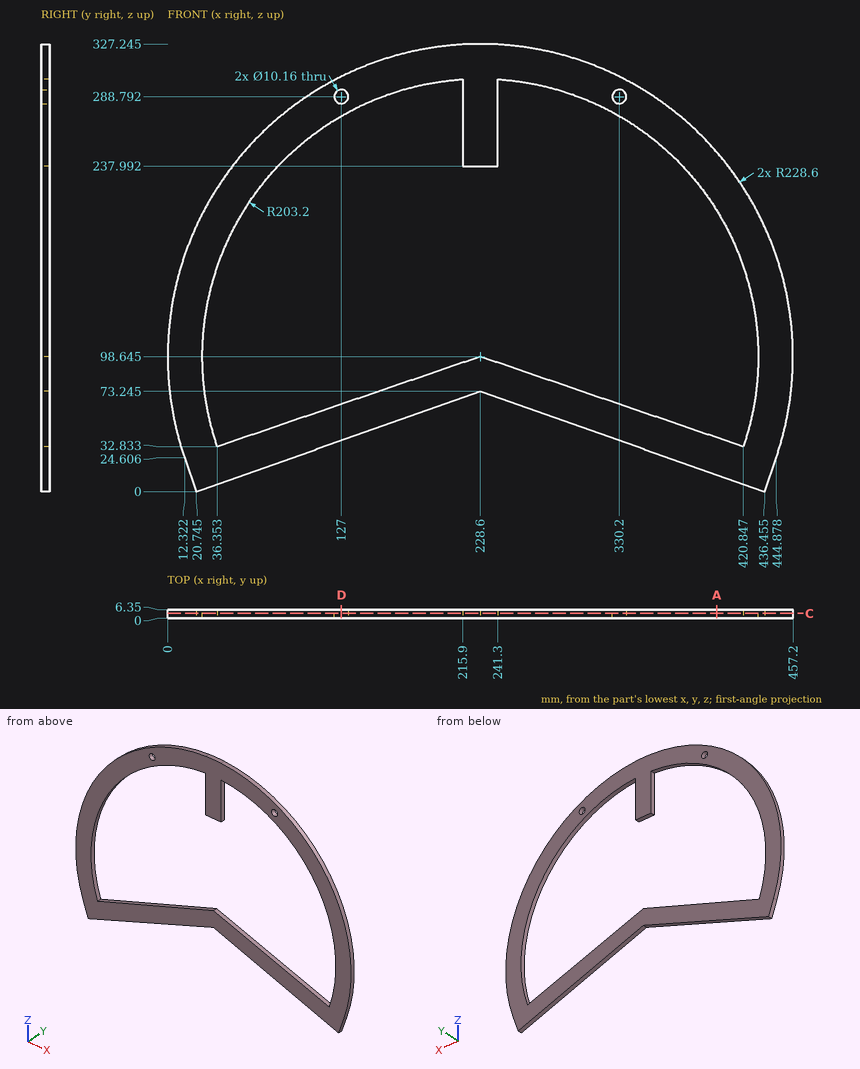
Answer from the drawing. Dimensions are ordinates in mm from the lowest x, y and z of the part. Give positions to 0.01 mm unless a question says otherwise; leave off trailing zeros. Order: outer loops, then holes, each group sorted by start corner. A loop starts at its lowest first (then second) coordinate and runs counter-clockwise, first axis right, second up.
(1) Straight lines are drawn through the part: L1, parallel to Z at x = 127, y = 4.75 (1 decimal); L2, parallel to X at y = 3, z = 236 (1 decimal); L3, parallel to Z at x = 186, y = 3.5 (1 decimal). For each, find the intervals that lie inside material, in ascending order.
(2) Find section A-A (x = 401.5). Give the vertices of the cut face in (y, z), plus the area to 3 significant figures.
(3) Find section C-C (y = 3.5). Give the vertices of the cut face in (x, z) (1 decimal).
(4) Find section D-D (x = 127). Give the number of separate pieces and of enclosed holes in the cut face, plus the area to 3 significant figures.
(5) Given pin 1 (9 mm diameter, centred on x = 127, z = 288.79, fed in from +Y); pin 2 (1.5 mm diameter, centred on x = 67.5, y = 2.5, fed in from -Z); pin 3 (11.5 mm diameter, centred on x = 330.2, z = 288.79, fed in from -Y); pin 4 (1 mm diameter, centred on x = 171, y = 2, fed in from -Z), each flat-ended and moving along its own axis, determine where each tip first touches the part or whether it passes through.
Result sheet:
1. L1: z = 37.4 to 63.9, 274.6 to 283.7, 293.9 to 303.4
1. L2: x = 45.9 to 78.9, 378.3 to 411.3
1. L3: z = 58.2 to 84.1, 297.3 to 323.2
2. outline: (0, 12.32) - (6.35, 12.32) - (6.35, 39.46) - (0, 39.46) - close; (0, 205.4) - (6.35, 205.4) - (6.35, 248.19) - (0, 248.19) - close
2. area: 444 mm2
3. outline: (12.3, 24.6) - (20.7, 0) - (228.6, 73.2) - (436.5, 0) - (444.9, 24.6) arc R228.6 ccw to (241.3, 326.9) arc R228.6 ccw to (215.9, 326.9) arc R228.6 ccw to start; hole (36.4, 32.8) - (228.6, 98.6) - (420.8, 32.8) arc R203.2 ccw to (241.3, 301.4) - (241.3, 238) - (215.9, 238) - (215.9, 301.4) arc R203.2 ccw to start; hole circle Ø10.2 at (127, 288.8); hole circle Ø10.2 at (330.2, 288.8)
4. separate pieces: 3
4. enclosed holes: 0
4. area: 286 mm2
5. pin 1: passes through
5. pin 2: stops at z = 16.21
5. pin 3: stops at y = 0
5. pin 4: stops at z = 52.77
